CAD build for the part. Positions are in the model's coordinates, mm. Round coordinates to 2 decimals unless told otherwise and drop trailing zeros. Write each loop counter-clockwise with the first axis right and the second up, starting at its lowest first coordinate (ties: lowest second). Pieces come first, ordered by that corner, then holes. Notation, with made-up numbers: (59.25, 46) - (90.25, 46) arc R20 ccw to (90.25, 68) - close; hole circle Ø8 at (16.5, 17). An arc over 180 degrees is marked (long way). Answer in a Markdown table with one row per item.
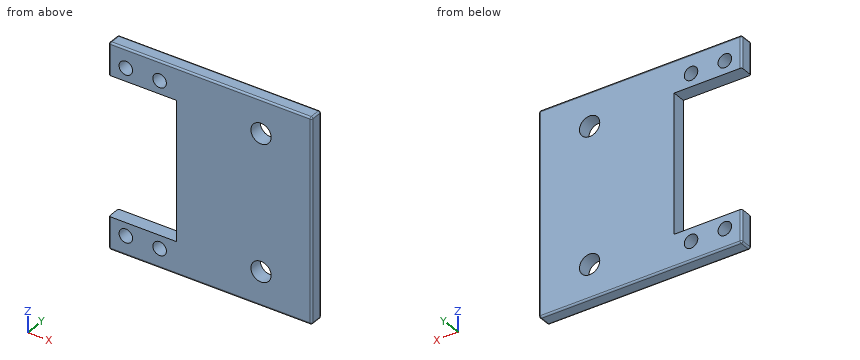
```python
from build123d import *

# Parameters (mm, degrees)
SKETCH1_R           = 2
SKETCH1_R_2         = 3
BOSS_EXTRUDE1_DEPTH = 2
FILLET1_R           = 0.5


with BuildPart() as part:
    # Sketch1 → Boss-Extrude1 (new, symmetric)
    with BuildSketch(Plane(origin=(0, 0, 0), x_dir=(1, 0, 0), z_dir=(0, 1, 0))):
        Polygon((-30, -20.45), (-30, -30), (30, -30), (30, 30), (-30, 30), (-30, 20.45), (-10, 20.45), (-10, -20.45), align=None)
        with Locations(Location((-25, -24.3, 0), (0, 0, 270))):
            Circle(SKETCH1_R, mode=Mode.SUBTRACT)
        with Locations(Location((-15, -24.3, 0), (0, 0, 270))):
            Circle(SKETCH1_R, mode=Mode.SUBTRACT)
        with Locations(Location((15, -20, 0), (0, 0, 270))):
            Circle(SKETCH1_R_2, mode=Mode.SUBTRACT)
        with Locations(Location((-25, 24.3, 0), (0, 0, 270))):
            Circle(SKETCH1_R, mode=Mode.SUBTRACT)
        with Locations(Location((-15, 24.3, 0), (0, 0, 270))):
            Circle(SKETCH1_R, mode=Mode.SUBTRACT)
        with Locations(Location((15, 20, 0), (0, 0, 270))):
            Circle(SKETCH1_R_2, mode=Mode.SUBTRACT)
    extrude(amount=BOSS_EXTRUDE1_DEPTH, both=True)

    # Fillet1
    fillet1_edges = [part.edges().sort_by_distance(p)[0] for p in [
        (-30, -2, -25.225),
        (0, -2, -30),
        (30, -2, 0),
        (0, -2, 30),
        (-30, -2, 25.225),
        (-30, 0, -30),
        (30, 0, -30),
        (30, 0, 30),
        (-30, 0, 30),
        (-30, 2, 25.225),
        (0, 2, 30),
        (30, 2, 0),
        (0, 2, -30),
        (-30, 2, -25.225),
    ]]
    fillet(fillet1_edges, radius=FILLET1_R)


solid = part.part
```
Q1. Saw through at B-B on y = 0.2. List the corners of the cut face in (x, z), then the cut area to 3 significant figures.
Computed:
| item | result |
|---|---|
| outline | (-30, -29.5) arc R0.5 ccw to (-29.5, -30) - (29.5, -30) arc R0.5 ccw to (30, -29.5) - (30, 29.5) arc R0.5 ccw to (29.5, 30) - (-29.5, 30) arc R0.5 ccw to (-30, 29.5) - (-30, 20.45) - (-10, 20.45) - (-10, -20.45) - (-30, -20.45) - close; hole circle Ø4 at (-25, -24.3); hole circle Ø4 at (-25, 24.3); hole circle Ø4 at (-15, -24.3); hole circle Ø4 at (-15, 24.3); hole circle Ø6 at (15, -20); hole circle Ø6 at (15, 20) |
| area | 2,670 mm2 |
Q2. Drill centre lines: line 1 (X direction, y = 0.5, z = 24.3); line 2 (Z direction, x = -15.5, y = -1.7); line 3 (Z direction, x = -24, y = 0.35). Where is each one in solid material? Low to high.
Computed:
| item | result |
|---|---|
| line 1 | x = -30 to -27, -23 to -17, -13 to 30 |
| line 2 | z = -29.96 to -26.24, -22.36 to -20.45, 20.45 to 22.36, 26.24 to 29.96 |
| line 3 | z = -30 to -26.03, -22.57 to -20.45, 20.45 to 22.57, 26.03 to 30 |
Q3. Flat gauge pin, fed straight in: pin 1 (2.5 mm diameter, centred on x = -25, z = 24.3, fed in from +Y). Where does the tip first touch, or does it go through?
Computed:
| item | result |
|---|---|
| pin 1 | passes through |
Q4. Saw through at D-D on z = 24.5. List the corners of the cut face in (x, y), then the cut area to 3 significant figures.
Computed:
| item | result |
|---|---|
| outline | (-30, -1.5) arc R0.5 ccw to (-29.5, -2) - (-26.99, -2) - (-26.99, 2) - (-29.5, 2) arc R0.5 ccw to (-30, 1.5) - close; (-23.01, -2) - (-16.99, -2) - (-16.99, 2) - (-23.01, 2) - close; (-13.01, -2) - (29.5, -2) arc R0.5 ccw to (30, -1.5) - (30, 1.5) arc R0.5 ccw to (29.5, 2) - (-13.01, 2) - close |
| area | 208 mm2 |
Q5. Saw through at A-A on x = 15. List the corners of the cut face in (y, z).
Computed:
| item | result |
|---|---|
| outline | (-2, -29.5) arc R0.5 ccw to (-1.5, -30) - (1.5, -30) arc R0.5 ccw to (2, -29.5) - (2, -23) - (-2, -23) - close; (-2, -17) - (2, -17) - (2, 17) - (-2, 17) - close; (-2, 23) - (2, 23) - (2, 29.5) arc R0.5 ccw to (1.5, 30) - (-1.5, 30) arc R0.5 ccw to (-2, 29.5) - close |
Q6. Saw through at C-C on x = -25. List the corners of the cut face in (y, z), then the cut area to 3 significant figures.
Computed:
| item | result |
|---|---|
| outline | (-2, -29.5) arc R0.5 ccw to (-1.5, -30) - (1.5, -30) arc R0.5 ccw to (2, -29.5) - (2, -26.3) - (-2, -26.3) - close; (-2, -22.3) - (2, -22.3) - (2, -20.45) - (-2, -20.45) - close; (-2, 20.45) - (2, 20.45) - (2, 22.3) - (-2, 22.3) - close; (-2, 26.3) - (2, 26.3) - (2, 29.5) arc R0.5 ccw to (1.5, 30) - (-1.5, 30) arc R0.5 ccw to (-2, 29.5) - close |
| area | 44.2 mm2 |
